Design review of the part shown in the three views and the two pictorial views. Dimensions are in mm from the part's minimum x, y and z. A direction names the side the tool comes from. Give positions to 0.01 mm unless a question says otherwise; leave off trailing zeros. Loops run counter-clockwise (first coordinate to the right, second up) from the corner with the lowest first, then second, coordinate; pieces in that order, holes last. Notation, with made-up numbers: (22.25, 17) -> (59.25, 17) arc R18 ccw to (59.25, 27) -> close; hole circle Ø8 at (12, 49). An arc over 180 degrees is marked (long way). Answer as CSV lines item,"result".
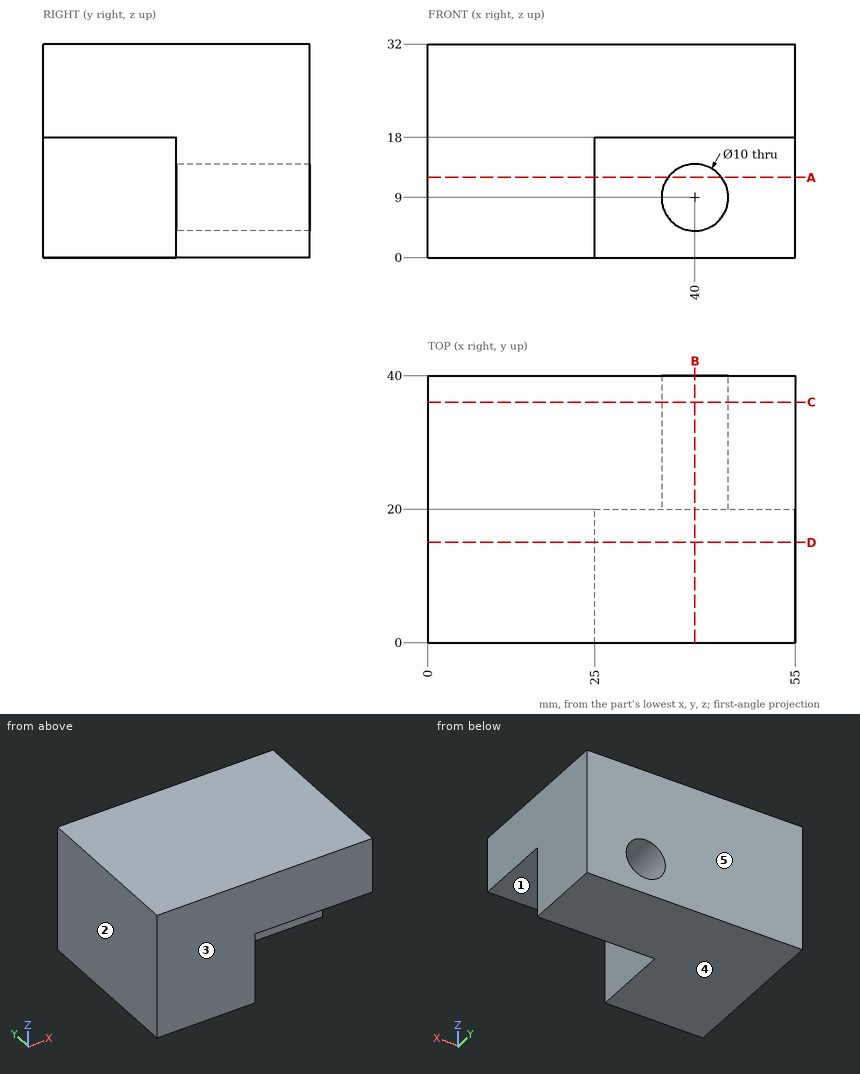
Q1. Clearance check with flat-ended pins moving along their axes: pin 1 Ø14.5 at (x, z) = (41.5, 5) entering from -Y; pin 2 Ø10 at (x, y) = (43.5, 13) entering from -Z; pin 3 Ø14.5 at (y, z) = (8, 6.5) entering from +X. State where each tip first meets the part, or that it passes through.
Filled sheet:
pin 1,"stops at y = 20"
pin 2,"stops at z = 18"
pin 3,"stops at x = 25"
Q2. We need section C-C, the plane y = 36. State the section outline as (x, z) points.
Filled sheet:
outline,"(0, 0) -> (55, 0) -> (55, 32) -> (0, 32) -> close; hole circle Ø10 at (40, 9)"
Q3. We need section D-D, the plane y = 15. State the section outline as (x, z) points, and give its area (3 significant figures).
Filled sheet:
outline,"(0, 0) -> (25, 0) -> (25, 18) -> (55, 18) -> (55, 32) -> (0, 32) -> close"
area,"1,220 mm^2"
Q4. To check wall thickness, follow probe 1 along Z at (x, y) = (40, 33.75); probe 2 along Z at (x, y) = (40, 16.5); probe 3 along X at (y, z) = (9, 12.5). State the ranges of each line that lie inside material, in increasing order. Write a range as from..to.
Filled sheet:
probe 1,"z = 0..4, 14..32"
probe 2,"z = 18..32"
probe 3,"x = 0..25"
Q5. We need section B-B, the plane x = 40. State the section outline as (y, z) points.
Filled sheet:
outline,"(0, 18) -> (20, 18) -> (20, 14) -> (40, 14) -> (40, 32) -> (0, 32) -> close; (20, 0) -> (40, 0) -> (40, 4) -> (20, 4) -> close"
Q6. The part is to be moulded in two halves that separate along Y. For the marked faces 3, 4 and 5, say which applies: pulls with the +Y half, pulls with the -Y half, needs draft (parallel to the pull), parting line crosses it, or undercut.
Filled sheet:
face 3,"pulls with the -Y half"
face 4,"needs draft"
face 5,"pulls with the +Y half"
Q7. For the marked faces 1 and 2, list the 3-axis set-ups (+Z, -Z, +X, -X, +Y, -Y) from which the entire face can be reached by the end or side of a thin tool; tool diameter is ignored.
Filled sheet:
face 1,"-Z, +X, -Y"
face 2,"+Z, -Z, -X, +Y, -Y"
Q8. We need section A-A, the plane z = 12. State the section outline as (x, y) points.
Filled sheet:
outline,"(0, 0) -> (25, 0) -> (25, 20) -> (36, 20) -> (36, 40) -> (0, 40) -> close; (44, 20) -> (55, 20) -> (55, 40) -> (44, 40) -> close"
